Could you check a few things on this model? Use its own coordinates, in mm. A direction names the side the tool comes from. Round coordinates to 2 decimals unless told otherwise and drop trailing zeros. Order: outer loops, then holes, each group sorted by start corner. A loop starts at its lowest first (then second) coordinate and runs counter-clockwise, first axis right, second up. Notation, with made-up numbers: (82.5, 77.25) - (98.5, 77.25) arc R20 cw to (98.5, 94.25) - close; hole circle Ø9 at (18.5, 45.25). An arc over 180 degrees is marked (long way). Use one line per item in the form item = value.
from build123d import *

# Parameters (mm, degrees)
F1_DEPTH      = 71
F1_DEPTH_BACK = 71
F2_W          = 194.8
F2_H          = 139.6
F3_DEPTH      = 49.62
F4_W          = 35.56
F4_H          = 7.62
F5_DEPTH      = 25
F6_W          = 5
F6_H          = 1.2
F7_DEPTH      = 5
F8_W          = 1.2
F8_H          = 48.42
F9_DEPTH      = 1.21
F10_W         = 5
F10_H         = 1.2
F11_DEPTH     = 5
F12_W         = 1.2
F12_H         = 48.42
F13_DEPTH     = 1.21
F15_DEPTH     = 1.2
F17_DEPTH     = 1.2
F18_W         = 5
F18_H         = 5
F19_DEPTH     = 1.2


with BuildPart() as f1:
    # F0 (on Front) → F1 (new body, two sides)
    with BuildSketch(Plane.XZ) as f1_sk:
        Polygon((98.6, 25.41), (0, 25.41), (-98.6, 25.41), (-98.6, -25.41), (0, -25.41), (98.6, -25.41), align=None)
    extrude(amount=F1_DEPTH)
    extrude(f1_sk.sketch, amount=-F1_DEPTH_BACK)

    # F2 (on face) → F3 (cut)
    with BuildSketch(Plane.XY.offset(25.41)):
        Rectangle(F2_W, F2_H)
    extrude(amount=-F3_DEPTH, mode=Mode.SUBTRACT)

    # F4 (on face) → F5 (cut)
    with BuildSketch(Plane(origin=(0, 71, 0), x_dir=(-1, 0, 0), z_dir=(0, 1, 0))):
        with Locations((60.82, 21.6)):
            Rectangle(F4_W, F4_H)
    extrude(amount=-F5_DEPTH, mode=Mode.SUBTRACT)

    # F6 (on face) → F7 (cut)
    with BuildSketch(Plane(origin=(-98.6, 0, 0), x_dir=(0, -1, 0), z_dir=(-1, 0, 0))):
        with Locations((-68.5, -23.61)):
            Rectangle(F6_W, F6_H)
        with Locations((68.5, -23.61)):
            Rectangle(F6_W, F6_H)
    extrude(amount=-F7_DEPTH, mode=Mode.SUBTRACT)

    # F8 (on face) → F9 (cut)
    with BuildSketch(Plane(origin=(-98.6, 0, 0), x_dir=(0, -1, 0), z_dir=(-1, 0, 0))):
        with Locations((-70.4, 1.2)):
            Rectangle(F8_W, F8_H)
        with Locations((70.4, 1.2)):
            Rectangle(F8_W, F8_H)
    extrude(amount=-F9_DEPTH, mode=Mode.SUBTRACT)

    # F10 (on face) → F11 (cut)
    with BuildSketch(Plane.YZ.offset(98.6)):
        with Locations((68.5, -23.61)):
            Rectangle(F10_W, F10_H)
        with Locations((-68.5, -23.61)):
            Rectangle(F10_W, F10_H)
    extrude(amount=-F11_DEPTH, mode=Mode.SUBTRACT)

    # F12 (on face) → F13 (cut)
    with BuildSketch(Plane.YZ.offset(98.6)):
        with Locations((-70.4, 1.2)):
            Rectangle(F12_W, F12_H)
        with Locations((70.4, 1.2)):
            Rectangle(F12_W, F12_H)
    extrude(amount=-F13_DEPTH, mode=Mode.SUBTRACT)

    # F14 (on face) → F15 (cut, through all)
    with BuildSketch(Plane(origin=(-98.6, 0, 0), x_dir=(0, -1, 0), z_dir=(-1, 0, 0))):
        Polygon((-56, 25.41), (-66, 25.41), (-69.8, 25.41), (-69.8, -23.01), (-66, -23.01), align=None)
        Polygon((69.8, 25.41), (66, 25.41), (56, 25.41), (66, -23.01), (69.8, -23.01), align=None)
    extrude(amount=-F15_DEPTH, mode=Mode.SUBTRACT)

    # F16 (on face) → F17 (cut, through all)
    with BuildSketch(Plane.YZ.offset(98.6)):
        Polygon((-56, 25.41), (-66, 25.41), (-69.8, 25.41), (-69.8, -23.01), (-66, -23.01), align=None)
        Polygon((66, -23.01), (69.8, -23.01), (69.8, 25.41), (56, 25.41), align=None)
    extrude(amount=-F17_DEPTH, mode=Mode.SUBTRACT)

    # F18 (on face) → F19 (cut, through all)
    with BuildSketch(Plane(origin=(0, 0, -25.41), x_dir=(1, 0, 0), z_dir=(0, 0, -1))):
        with Locations((-96.1, -68.5)):
            Rectangle(F18_W, F18_H)
        with Locations((96.1, -68.5)):
            Rectangle(F18_W, F18_H)
        with Locations((96.1, 68.5)):
            Rectangle(F18_W, F18_H)
        with Locations((-96.1, 68.5)):
            Rectangle(F18_W, F18_H)
    extrude(amount=-F19_DEPTH, mode=Mode.SUBTRACT)


solid = f1.part
Item 1: Imagine slicing it at D-D on z = 20. Please give me the cut outline in (x, y), plus the area to 3 significant figures.
Found:
outline = (-98.6, -57.12) - (-97.4, -57.12) - (-97.4, 57.12) - (-98.6, 57.12) - close; (-97.39, -71) - (97.39, -71) - (97.39, -69.8) - (-97.39, -69.8) - close; (-97.39, 69.8) - (-78.6, 69.8) - (-78.6, 71) - (-97.39, 71) - close; (-43.04, 69.8) - (97.39, 69.8) - (97.39, 71) - (-43.04, 71) - close; (97.4, -57.12) - (98.6, -57.12) - (98.6, 57.12) - (97.4, 57.12) - close
area = 699 mm2
Item 2: Will these pins go through, and if not, where does the flat tip stop? P1, Ø1.9, axis at y = -68.5, z = -23.5, coming from the +X side; P2, Ø1.3, axis at y = -70.5, z = 11, coming from the -X side; P3, Ø3, axis at x = 43, y = -48.5, coming from the +Z side.
Found:
P1 = 93.6
P2 = -97.39
P3 = -24.21
Item 3: Imagine slicing it at A-A on z = 7.5. Please give me the cut outline in (x, y), plus the area to 3 significant figures.
Found:
outline = (-98.6, -59.7) - (-97.4, -59.7) - (-97.4, 59.7) - (-98.6, 59.7) - close; (-97.39, -71) - (97.39, -71) - (97.39, -69.8) - (-97.39, -69.8) - close; (-97.39, 69.8) - (97.39, 69.8) - (97.39, 71) - (-97.39, 71) - close; (97.4, -59.7) - (98.6, -59.7) - (98.6, 59.7) - (97.4, 59.7) - close
area = 754 mm2
Item 4: If we mould it in two halves opening along X, with no side actions, what happens to faces 4 (the face through (-97.4, -1, 1)), 5 (the face through (97.4, -1, 1)), 6 (the face through (-1, 69.8, 1)), 7 (the face through (98.6, -1, 0))? For each: released by +X, released by -X, zero draft, split by the parting line, or undercut.
Found:
face_4 = undercut
face_5 = undercut
face_6 = zero draft
face_7 = released by +X
Item 5: For faces 1 (the face through (-1, 1, -24.21)), 2 (the face through (-1, -69.8, 1)), 3 (the face through (-98.6, -1, 0)), which set-ups out of +Z, -Z, +X, -X, +Y, -Y let a thin tool reach every point of the face, with its end or its side?
Found:
face_1 = +Z
face_2 = +Z, +X, -X
face_3 = +Z, -Z, -X, +Y, -Y
Item 6: Imagine slicing it at B-B on y = 35. Please give me the cut outline in (x, z).
Found:
outline = (-98.6, -25.41) - (98.6, -25.41) - (98.6, 25.41) - (97.4, 25.41) - (97.4, -24.21) - (-97.4, -24.21) - (-97.4, 25.41) - (-98.6, 25.41) - close
Item 7: I need wall thicknesses on L1, parallel to X at y = 51, z = 5; L2, parallel to Y at x = 86, z = 8; L3, parallel to Z at x = -77, y = 12.5. Which ranges of each line are inside material? Lowest first, please.
Found:
L1 = -98.6 to -97.4, 97.4 to 98.6
L2 = -71 to -69.8, 69.8 to 71
L3 = -25.41 to -24.21
Item 8: Imagine slicing it at C-C on x = 82. Please give me the cut outline in (y, z), plus the area to 3 significant figures.
Found:
outline = (-71, -25.41) - (71, -25.41) - (71, 25.41) - (69.8, 25.41) - (69.8, -24.21) - (-69.8, -24.21) - (-69.8, 25.41) - (-71, 25.41) - close
area = 289 mm2
